The model under review builds one solid part; all positions refer to its coordinate system, in mm. A direction names the side the tool comes from. Coordinates: 2 decimals unless noted, no trailing zeros. Loops run counter-clockwise (first coordinate to the right, second up) from the corner with the lowest first, then second, coordinate; pieces in that order, holes last. Notation, with made-up numbers: M 81.25,60 L 130.25,60 A20 ccw 130.25,91 Z; hole C -30.5,-3.75 d8. An arc over 180 degrees is marked long. Use one line per item in the form item = value.
Autodesk Inventor part; units mm, degrees
ref_plane "YZ Plane" through (0, 0, 0) normal (1, 0, 0) x (0, 1, 0)
ref_plane "XZ Plane" through (0, 0, 0) normal (0, 1, 0) x (-1, 0, 0)
ref_plane "XY Plane" through (0, 0, 0) normal (0, 0, 1) x (1, 0, 0)
sketch "Sketch1" plane through (0, 0, 0) normal (0, 1, 0) x (-1, 0, 0)
  circle A0 centre (0, 0) radius 2.85
  circle A1 centre (0, 0) radius 4.85
  dimension "d0" = 5.7
  dimension "d1" = 2
extrude "Extrusion1" add sketch "Sketch1" along normal blind 10
sketch "Sketch2" plane through (0, 0, 0) normal (1, 0, 0) x (0, 1, 0)
  circle A0 centre (7, 6.85) radius 2
  circle A1 centre (7, 6.85) radius 4.5
  line L0 (10, -4.85) -> (10, 4.85)
  line L1 (0, -4.85) -> (0, 4.85)
  line L2 (0, 4.85) -> (10, 4.85)
  point P0 (0, 0)
  dimension "d4" = 4
  dimension "d5" = 9
  dimension "d6" = 7
extrude "Extrusion2" add sketch "Sketch2" along normal mid plane 4
sketch "Sketch3" plane through (0, 0, 0) normal (0, -1, 0) x (1, 0, 0)
  circle A0 centre (0, 0) radius 4.85
  circle A1 centre (0, 0) radius 2.85
extrude "Extrusion3" add sketch "Sketch3" along normal blind 3 contours A0 | A1
fillet "Fillet1" radius 2 1 edges at (-4.85, -3, 0)
extrude "Extrusion4" cut sketch "Sketch1" along normal blind 100 contours A0
properties part number "Landing_leg_shoe"
1. The part is to be moulded in two halves that separate along X. For faces 3 (the face through (0, 0, 0)), 4 (the face through (-2, 7, 9)), 5 (the face through (0, 5, 6.9)), say which applies: pulls with the +X half, pulls with the -X half, needs draft (parallel to the pull), parting line crosses it, or undercut.
Response values:
face_3 = undercut
face_4 = pulls with the -X half
face_5 = needs draft
2. Machinability: for faces 1 (the face through (2.262, 4.93, 1.734)), 2 (the face through (0, -3, 0)), which of the approach directions +Z, -Z, +X, -X, +Y, -Y give a long, thin tool a straight path to every point of the face, cutting with its end or side? Answer none if there is none.
Response values:
face_1 = +Y
face_2 = +Z, -Z, +X, -X, -Y
3. Add section B-B (z = 6.85). State the section outline as (x, y) points.
Response values:
outline = M -2,2.5 L 2,2.5 L 2,5 L -2,5 Z; M -2,9 L 2,9 L 2,11.5 L -2,11.5 Z
4. Add section C-C (y = 2). State the section outline as (x, z) points, then the cut area to 3 significant figures.
Response values:
outline = C 0,0 d9.7; hole C 0,0 d5.7
area = 48.4 mm^2
5. Add section D-D (z = 0). State the section outline as (x, y) points.
Response values:
outline = M -4.85,-1 A2 ccw -2.85,-3 L 2.85,-3 A2 ccw 4.85,-1 L 4.85,10 L 2.85,10 L 2.85,0 L -2.85,0 L -2.85,10 L -4.85,10 Z
6. Insertion check: P1, Ø1.5, axis at x = -3, y = 4.5, coming from the +Z side; P2, Ø1, axis at x = 2.5, y = 6, coming from the -Z side; P3, Ø4.5, axis at x = -0.5, z = 1, coming from the +Y side. Each pin has a flat end and moves straight along its axis. Give the tip position at first contact, or say it passes through.
Response values:
P1 = 4.3
P2 = -4.42
P3 = 10
7. Wall thickness on line 1 along Z through (x, y) = (0, 1.5); line 2 along Z through (x, y) = (-0.65, 7); line 3 along Y through (x, z) = (0.3, 6.85): over which ranges is each line inside the solid? List them lowest first. Write a range as from..to.
Response values:
line_1 = -4.85..-2.85, 2.85..4.85
line_2 = -4.81..-2.77, 2.77..4.85, 8.85..11.35
line_3 = 2.5..5, 9..11.5
8. Add section A-A (y = 7). State the section outline as (x, z) points, then the cut area to 3 significant figures.
Response values:
outline = M -2,4.42 A4.85 ccw long 2,4.42 L 2,4.85 L -2,4.85 Z; M -2,8.85 L 2,8.85 L 2,11.35 L -2,11.35 Z; hole C 0,0 d5.7
area = 58.9 mm^2
